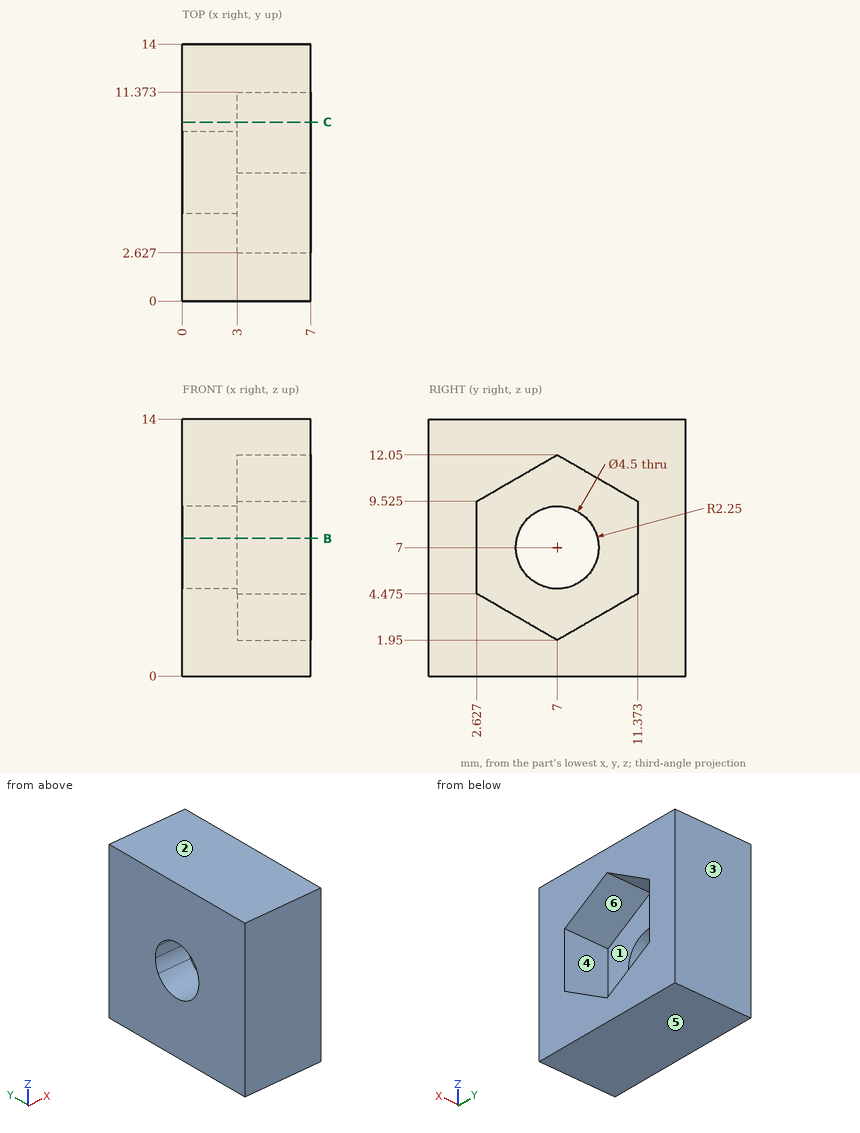
The drawing under review shows one solid part. Ordinate dimensions are in mm from its lowest x, y, z. A direction names the side the tool comes from. Coordinates: 2 decimals unless noted, no trailing zeros. Write each loop counter-clockwise with the first axis right and the second up, starting at its lowest first coordinate (ties: lowest second). Pieces come first, ordered by that corner, then holes. Notation, with made-up numbers: (79.5, 40) -> (85.5, 40) arc R25 cw to (85.5, 74) -> close; hole circle Ø10 at (88.25, 84). An arc over 180 degrees is marked (long way). Write each question's results on one line, items separated by ' | '. Start each with the question number.
1) Consider section C-C (y = 9.75). Write out the cut boundary in (x, z).
2) Wall thickness on L1, parallel to Z at x = 1.4, y = 7; L2, parallel to Y at x = 5, z = 6.5: over which ranges is each line inside the solid? List them lowest first. Write a range as [from, to].
3) Consider section B-B (z = 7.5). Write out the cut boundary in (x, y).
4) The part is to be moulded in two halves that separate along Z. For the marked faces 1, 2, 3 and 4, say which applies: +Z half, -Z half, draft (parallel to the pull), parting line (faces both ways), or undercut.
5) For the marked faces 5 and 6, list the 3-axis set-ups (+Z, -Z, +X, -X, +Y, -Y) from which the entire face can be reached by the end or side of a thin tool; tool diameter is ignored.
Geometry says:
1) outline: (0, 0) -> (7, 0) -> (7, 3.54) -> (3, 3.54) -> (3, 10.46) -> (7, 10.46) -> (7, 14) -> (0, 14) -> close
2) L1: [0, 4.75], [9.25, 14] | L2: [0, 2.63], [11.37, 14]
3) outline: (0, 0) -> (7, 0) -> (7, 2.63) -> (3, 2.63) -> (3, 4.81) -> (0, 4.81) -> close; (0, 9.19) -> (3, 9.19) -> (3, 11.37) -> (7, 11.37) -> (7, 14) -> (0, 14) -> close
4) face 1: undercut | face 2: +Z half | face 3: draft | face 4: undercut
5) face 5: -Z, +X, -X, +Y, -Y | face 6: +X
